Print and shaded views of the part. All mm, measured from the part's lowest x, y and z. A direction names the side the tool comes from. Coordinates: 2 decimals unless noted, no trailing zeros. Write each loop counter-clockwise with the first axis right and the second up, starting at its lowest first coordinate (ties: lowest second). Pieces come first, ordered by that corner, then holes. Notation, with made-up numbers: (-30, 52) -> (7, 52) arc R21 ccw to (7, 65) -> close; hole circle Ø4 at (-2, -13.5). An arc over 180 degrees is marked (long way). Write item = value, one per line.
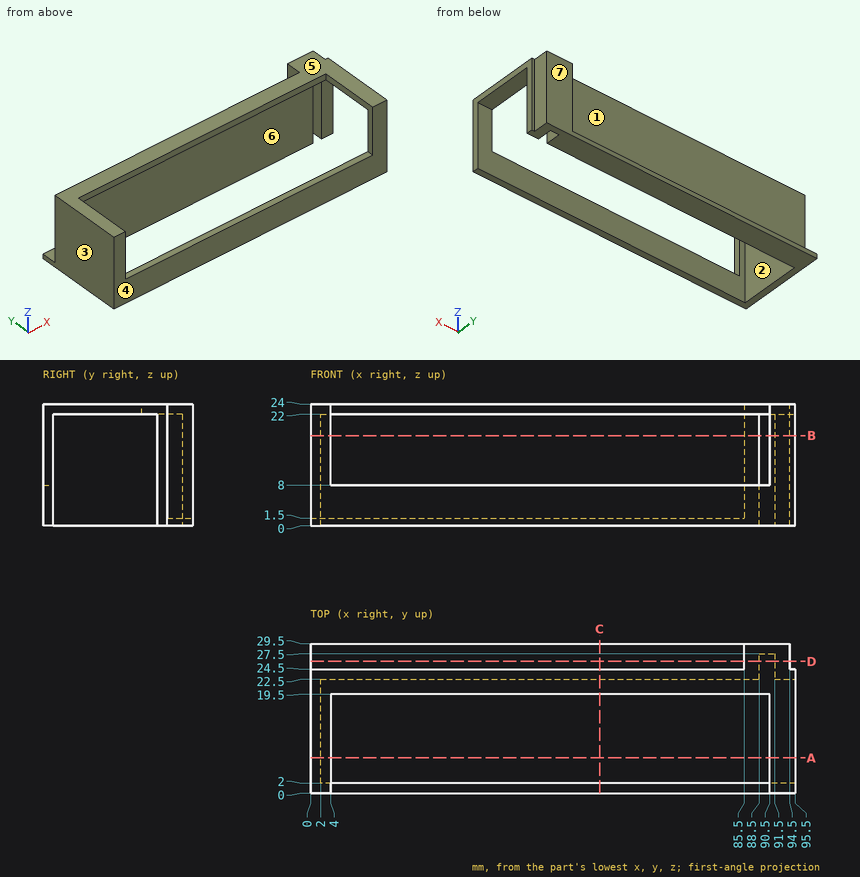
Q1. Saw through at D-D on y = 26. Give the cut face in (x, z).
Model answer:
outline = (0, 0) -> (88.5, 0) -> (88.5, 22) -> (91.5, 22) -> (91.5, 0) -> (94.5, 0) -> (94.5, 24) -> (85.5, 24) -> (85.5, 1.5) -> (0, 1.5) -> close
Q2. Which spindle directions (+Z, -Z, +X, -X, +Y, -Y) get a long thin tool onto all of the face, cutting with end or side? Do the marked faces 1, 2 and 3. Say none if no direction does.
Model answer:
face_1 = +Z, -X, +Y
face_2 = -Z, +X
face_3 = +Z, -Z, -X, +Y, -Y
Q3. Saw through at A-A on y = 7. Give the cut face in (x, z), and give its area (3 significant figures).
Model answer:
outline = (0, 0) -> (2, 0) -> (2, 22) -> (4, 22) -> (4, 24) -> (0, 24) -> close; (90.5, 22) -> (95.5, 22) -> (95.5, 24) -> (90.5, 24) -> close
area = 62.0 mm²
Q4. Probe line 1 (X direction, y = 23.25, z = 18.75); line 2 (Y direction, x = 18.5, z = 1); line 3 (Y direction, x = 87, z = 9). List the from-to ranges inside material, lowest first. Write a range as from..to.
Model answer:
line_1 = 0..88.5, 91.5..95.5
line_2 = 0..2, 22.5..29.5
line_3 = 22.5..29.5
Q5. Mould opens along Y. For the marked faces 4, 5, 6 and 7 say: released by +Y, released by -Y, zero draft, split by the parting line, or undercut.
Model answer:
face_4 = released by -Y
face_5 = zero draft
face_6 = undercut
face_7 = released by +Y
Q6. Pin check, flat tips, straight feed: pin 1 (11 mm diameter, centred on x = 28, z = 10, fed in from +Y); pin 2 (1 mm diameter, centred on y = 7.5, z = 3.5, fed in from +X); pin 3 (2 mm diameter, centred on x = 42, y = 1, fed in from +Z). Stop position of each tip, or through.
Model answer:
pin_1 = 24.5
pin_2 = 2
pin_3 = 8
Q7. Saw through at B-B on z = 17.75. Give the cut face in (x, y), and give its area (3 significant figures).
Model answer:
outline = (0, 0) -> (4, 0) -> (4, 2) -> (2, 2) -> (2, 22.5) -> (88.5, 22.5) -> (88.5, 27.5) -> (91.5, 27.5) -> (91.5, 22.5) -> (95.5, 22.5) -> (95.5, 24.5) -> (94.5, 24.5) -> (94.5, 29.5) -> (85.5, 29.5) -> (85.5, 24.5) -> (0, 24.5) -> close; (90.5, 0) -> (95.5, 0) -> (95.5, 2) -> (90.5, 2) -> close
area = 280 mm²
Q8. Saw through at C-C on x = 57. Give the cut face in (y, z).
Model answer:
outline = (0, 0) -> (2, 0) -> (2, 8) -> (0, 8) -> close; (19.5, 22) -> (22.5, 22) -> (22.5, 0) -> (29.5, 0) -> (29.5, 1.5) -> (24.5, 1.5) -> (24.5, 24) -> (19.5, 24) -> close
